from build123d import *

# Parameters (mm, degrees)
SKETCH1_R           = 2.5
BOSS_EXTRUDE1_DEPTH = 3.048


with BuildPart() as part:
    # Sketch1 → Boss-Extrude1 (new body)
    with BuildSketch(Plane.XY):
        with BuildLine():
            Line((0, 0), (71.622808257, 52.037016174))
            Line((71.622808257, 52.037016174), (88.501669832, 28.805256264))
            add(Edge.make_bspline(
                [(88.501669832, 28.805256264), (92.966978859, 22.659285651), (98.410551954, 17.410609678), (104.704030367, 13.341863973)],
                knots=[0.5, 0.5, 0.5, 0.5, 0.915853648, 0.915853648, 0.915853648, 0.915853648], degree=3))
            Line((104.704030367, 13.341863973), (104.658496812, 13.271443843))
            ThreePointArc((104.658496812, 13.271443843), (119.335898328, 9.736398283), (110.087731709, 21.669297201))
            add(Edge.make_bspline(
                [(96.52401812, 34.63383347), (97.463660016, 33.340527353), (99.467318776, 30.820691276), (103.81543362, 26.262690934), (107.476268967, 23.357612806), (110.087731709, 21.669297201)],
                knots=[0.5, 0.5, 0.5, 0.5, 0.603963412, 0.707926824, 0.915853648, 0.915853648, 0.915853648, 0.915853648], degree=3))
            Line((96.52401812, 34.63383347), (82.711847228, 53.644655768))
            Line((82.711847228, 53.644655768), (82.711847228, 60.093674581))
            Line((82.711847228, 60.093674581), (113.262379212, 82.289935321))
            Line((113.262379212, 82.289935321), (107.38452669, 90.380105265))
            Line((107.38452669, 90.380105265), (82.711847228, 72.454354356))
            Line((82.711847228, 72.454354356), (-5.877852523, 72.454354356))
            Line((-5.877852523, 72.454354356), (-65.877852523, 72.454354356))
            Line((-65.877852523, 72.454354356), (-65.877852523, 62.454354356))
            Line((-65.877852523, 62.454354356), (-43.945146495, 62.454354356))
            Line((-43.945146495, 62.454354356), (-66.676672481, 0))
            Line((-66.676672481, 0), (-57.279746273, -3.420201433))
            Line((-57.279746273, -3.420201433), (-9.396926208, -3.420201433))
            Line((-9.396926208, -3.420201433), (0, 0))
        make_face()
        with Locations((112.61759651, 14.07979857)):
            Circle(SKETCH1_R, mode=Mode.SUBTRACT)
        Polygon((-3.558033622, 9.775617033), (68.948028023, 62.454354356), (-5.877852523, 62.454354356), (-22.731525986, 62.454354356), align=None, mode=Mode.SUBTRACT)
        Polygon((-13.036628551, 6.579798567), (-33.338336241, 62.358282022), (-53.640043931, 6.579798567), align=None, mode=Mode.SUBTRACT)
    extrude(amount=BOSS_EXTRUDE1_DEPTH)


solid = part.part
Geometry: final body of the model. Coordinates: model frame, mm. A direction names the side the tool comes from. Give positions to 0.01 mm unless a question says otherwise; leave off trailing zeros. Loops run counter-clockwise (first coordinate to the right, second up) from the corner with the lowest first, then second, coordinate; pieces in that order, holes last. Notation, with made-up numbers: (-36, -4) - (14, -4) arc R36 ccw to (14, 33) - close; hole circle Ø4 at (84, 7). An arc over 180 degrees is marked (long way). Answer as CSV lines item,"result". Start each with the question number.
1. Section C-C, the plane z = 0.95. Give the number of separate pieces and of enclosed holes in the cut face, plus the area to 3 significant figures.
2. Section D-D, the plane y = 78.5. Return loops of the section in (x, z).
3. Reachability of faces 4 (the face through (-55.152, 31.664, 1.503)), 5 (the face through (79.944, 40.584, 1.503)), 6 (the face through (89.71, 44.01, 1.5)), 7 (the face through (-13.279, 36.484, 1.503)), 8 (the face through (-4.764, -1.734, 1.503)) from +Z, -Z, +X, -X, +Y, -Y: full face, straight path, thin tool, end or side. Return the list, or none.
4. Section B-B, the plane x = 2. Return loops of the section in (y, z).
5. Section A-A, the plane y = 37. Return loops of the section in (x, z), plus the area to 3 significant figures.
6. Ray query, L1, parallel to X at y = 43.5, z = 1.6; L2, parallel to X at y = 21.5, z = 0.45; L3, parallel to X at y = 8, z = 2. Return the intervals inside material, ascending.
7. Draft query along Y for faces 1 (the face through (97.773, 71.036, 1.503)), 2 (the face through (35.31, 25.654, 1.503)), 3 (the face through (110.365, 86.278, 1.503)). Return one class per face: released by +Y, released by -Y, zero draft, split by the parting line, or undercut.
8. Pin query (flat end, axial travel): P1, Ø1.5, axis at x = 24.5, z = 2, coming from the +Y side; P2, Ø1.5, axis at y = 56, z = 1, coming from the +X side; P3, Ø1.5, axis at y = 52.5, z = 1, coming from the +X side; P4, Ø4, axis at x = 112.62, y = 14.08, coming from the -Z side. Return the tip coordinate at first contact, or that it passes through.
Answers:
1,separate pieces,"1"
1,enclosed holes,"3"
1,area,"5,280 mm2"
2,outline,"(91.03, 0) - (108.05, 0) - (108.05, 3.05) - (91.03, 3.05) - close"
3,face 4,"+Z, -Z, -X"
3,face 5,"+Z, -Z, -Y"
3,face 6,"+Z, -Z, +X"
3,face 7,"+Z, -Z"
3,face 8,"+Z, -Z, +X, -Y"
4,outline,"(1.45, 0) - (13.81, 0) - (13.81, 3.05) - (1.45, 3.05) - close; (62.45, 0) - (72.45, 0) - (72.45, 3.05) - (62.45, 3.05) - close"
5,outline,"(-53.21, 0) - (-42.57, 0) - (-42.57, 3.05) - (-53.21, 3.05) - close; (-24.11, 0) - (-13.47, 0) - (-13.47, 3.05) - (-24.11, 3.05) - close; (33.91, 0) - (50.93, 0) - (50.93, 3.05) - (33.91, 3.05) - close; (82.55, 0) - (94.8, 0) - (94.8, 3.05) - (82.55, 3.05) - close"
5,area,"154 mm2"
6,L1,"x = -50.84 to -40.2, -26.47 to -15.83, 42.86 to 59.87, 77.83 to 90.08"
6,L2,"x = -58.85 to -48.21, -18.47 to -7.83, 12.58 to 29.59, 94.69 to 115.61"
6,L3,"x = -63.76 to -53.12, -13.55 to 11.01, 107.42 to 117.82"
7,face 1,"undercut"
7,face 2,"released by -Y"
7,face 3,"released by +Y"
8,P1,"stops at y = 72.45"
8,P2,"stops at x = 82.71"
8,P3,"stops at x = 84.09"
8,P4,"passes through"
